Work out the finished part from the listing and answer in its coordinate system (mm). Give positions to 0.01 mm unless a question says otherwise; leave off trailing zeros. Order: outer loops, then holes, each group sorted by start corner. A loop starts at its lowest first (then second) coordinate and runs counter-clockwise, first axis right, second up.
Autodesk Inventor part; units mm, degrees
ref_plane "YZ Plane" through (0, 0, 0) normal (1, 0, 0) x (0, 1, 0)
ref_plane "XZ Plane" through (0, 0, 0) normal (0, 1, 0) x (-1, 0, 0)
ref_plane "XY Plane" through (0, 0, 0) normal (0, 0, 1) x (1, 0, 0)
sketch "Sketch1" plane through (0, 0, 0) normal (0, 1, 0) x (-1, 0, 0)
  line L0 (0, 0) -> (25.4, 0)
  line L1 (25.4, 0) -> (25.4, -25.4)
  line L2 (25.4, -25.4) -> (0, -25.4)
  line L3 (0, -25.4) -> (0, 0)
  dimension "d0" = 25.4
  dimension "d1" = 25.4
extrude "Extrusion1" add sketch "Sketch1" along normal blind 50.8
sketch "Sketch2" plane through (-25.4, 0, 0) normal (0, 0, 1) x (1, 0, 0)
  circle A0 centre (12.7, 25.4) radius 6.35
  line L0 (25.4, 0) -> (25.4, 50.8)
  line L1 (0, 50.8) -> (25.4, 50.8)
  line L2 (25.4, 0) -> (0, 0)
  point P0 (12.7, 41.275)
  point P1 (12.7, 9.525)
  dimension "d4" = 12.7
  dimension "d5" = 12.7
  dimension "d6" = 25.4
  dimension "d7" = 9.525
  dimension "d8" = 9.525
hole "Hole1" at (-12.7, 41.275, 0) at (-12.7, 9.525, 0) direction (0, 0, -1) diameter 2.4892 end through all
sketch "Sketch3" plane through (-25.4, 0, 0) normal (0, 0, 1) x (1, 0, 0)
  circle A0 centre (12.7, 25.4) radius 6.35
  line L0 (0, 50.8) -> (25.4, 50.8)
  line L1 (0, 0) -> (0, 50.8)
  point P0 (25.4, 0)
  dimension "d16" = 12.7
  dimension "d17" = 25.4
  dimension "d18" = 12.7
extrude "Extrusion2" cut sketch "Sketch3" against normal through all
sketch "Sketch4" plane through (0, 50.8, 0) normal (0, 1, 0) x (1, 0, 0)
  line L0 (0, 0) -> (0, 25.4)
  line L1 (0, 25.4) -> (-25.4, 25.4)
  point P0 (-12.7, 12.7)
  dimension "d21" = 12.7
  dimension "d22" = 12.7
hole "Hole2" at (-12.7, 50.8, -12.7) direction (0, -1, 0) diameter 2.4892 end through all
sketch "Sketch5" plane through (0, 0, 0) normal (1, 0, 0) x (0, 0, -1)
  line L0 (25.4, 0) -> (25.4, 50.8)
  line L1 (25.4, 0) -> (0, 0)
  line L2 (0, 50.8) -> (25.4, 50.8)
  point P0 (12.7, 44.45)
  point P1 (12.7, 6.35)
  dimension "d30" = 12.7
  dimension "d31" = 12.7
  dimension "d32" = 6.35
  dimension "d33" = 6.35
hole "Hole3" at (0, 44.45, -12.7) at (0, 6.35, -12.7) direction (-1, 0, 0) diameter 2.4892 end through all
chamfer "Chamfer1" distance 1.27 angle 45 4 edges at (0, 50.8, -12.7) (-25.4, 50.8, -12.7) (0, 0, -12.7) (-25.4, 0, -12.7)
properties part number "chain and tube block"
1. The part is cut by section B-B (z = -17). Write down the section's boundary in (x, y) (3 decimals).
Findings below:
outline: (-25.4, 1.27) - (-24.13, 0) - (-1.27, 0) - (0, 1.27) - (0, 49.53) - (-1.27, 50.8) - (-24.13, 50.8) - (-25.4, 49.53) - close; hole circle Ø12.7 at (-12.7, 25.4); hole circle Ø2.489 at (-12.7, 9.525); hole circle Ø2.489 at (-12.7, 41.275)
2. The mould has two halves that part along X. Classify faces 1 (the face through (-9.77, 19.766, -12.522)), 2 (the face through (-10, 50.8, -13)), 3 (the face through (-0.64, 0.63, -12.52)): pulls with the +X half, pulls with the -X half, needs draft (parallel to the pull), parting line crosses it, or undercut.
Findings below:
face 1: undercut
face 2: needs draft
face 3: pulls with the +X half
3. The part is cut by section A-A (x = -17.75). Write down the section's boundary in (y, z), then the cut area to 3 significant figures.
Findings below:
outline: (0, -25.4) - (21.55, -25.4) - (21.55, 0) - (0, 0) - close; (29.25, -25.4) - (50.8, -25.4) - (50.8, 0) - (29.25, 0) - close; hole circle Ø2.49 at (6.35, -12.7); hole circle Ø2.49 at (44.45, -12.7)
area: 1,090 mm2
4. The part is cut by section C-C (y = 25.4). Write down the section's boundary in (x, z), then the cut area to 3 significant figures.
Findings below:
outline: (-25.4, -25.4) - (-19.05, -25.4) - (-19.05, 0) - (-25.4, 0) - close; (-6.35, -25.4) - (0, -25.4) - (0, 0) - (-6.35, 0) - close
area: 323 mm2
5. Straight lines are drawn through the part: probe 1 along Y at (x, z) = (-21.5, -12.7); probe 2 along Y at (x, z) = (-12.7, -8); probe 3 along Z at (x, y) = (-19.25, 44.5). For each, find the intervals that lie inside material, in ascending order.
Findings below:
probe 1: y = 0 to 5.11, 7.59 to 43.21, 45.69 to 50.8
probe 2: y = 0 to 8.28, 10.77 to 19.05, 31.75 to 40.03, 42.52 to 50.8
probe 3: z = -25.4 to -13.94, -11.46 to 0
